from build123d import *

# Parameters (mm, degrees)
ESQUISSE1_W        = 40.5
ESQUISSE1_H        = 33.5
ESQUISSE1_W_2      = 37.5
ESQUISSE1_H_2      = 30.5
BOSS_EXTRU_1_DEPTH = 4.5
ESQUISSE2_W        = 40.5
ESQUISSE2_H        = 33.5
BOSS_EXTRU_2_DEPTH = 1.5
ESQUISSE3_R        = 1.25
BOSS_EXTRU_3_DEPTH = 5


with BuildPart() as part:
    # Esquisse1 → Boss.-Extru.1 (new body)
    with BuildSketch(Plane(origin=(0, 0, 0), x_dir=(1, 0, 0), z_dir=(0, 1, 0))):
        with Locations((18.75, 15.25)):
            Rectangle(ESQUISSE1_W, ESQUISSE1_H)
        with Locations((18.75, 15.25)):
            Rectangle(ESQUISSE1_W_2, ESQUISSE1_H_2, mode=Mode.SUBTRACT)
    extrude(amount=BOSS_EXTRU_1_DEPTH)

    # Esquisse2 → Boss.-Extru.2 (add)
    with BuildSketch(Plane.XZ):
        with Locations((18.75, -15.25)):
            Rectangle(ESQUISSE2_W, ESQUISSE2_H)
    extrude(amount=BOSS_EXTRU_2_DEPTH)

    # Esquisse3 → Boss.-Extru.3 (add)
    with BuildSketch(Plane(origin=(0, 0, 0), x_dir=(1, 0, 0), z_dir=(0, 1, 0))):
        with Locations(Location((18.75, 26.75, 0), (0, 0, 90))):
            Circle(ESQUISSE3_R)
        with Locations(Location((18.75, 3.75, 0), (0, 0, 90))):
            Circle(ESQUISSE3_R)
    extrude(amount=BOSS_EXTRU_3_DEPTH)


solid = part.part
Could you check a few things on this model? Use its own coordinates, in mm. A direction names the side the tool comes from. Coordinates: 2 decimals unless noted, no trailing zeros. Order: outer loops, then holes, each group sorted by start corner. A loop starts at its lowest first (then second) coordinate and runs counter-clockwise, first axis right, second up. Notation, with made-up numbers: (-19.75, 37.25) -> (36.25, 37.25) arc R24 ccw to (36.25, 57.25) -> close; hole circle Ø1 at (3.5, -29). An arc over 180 degrees is marked (long way). One line per item, written item: value. Start each with the question number.
1) We'd pull the mould along X, two halves only. Please class faces 3 (the flat face through (18, 2, 1.5)), 4 (the flat face through (39, 2, -15)), 5 (the cylindrical face through (19.97, 2.46, -3.48)): +X half, -X half, draft (parallel to the pull), parting line (faces both ways), or undercut.
2) Imagine slicing it at A-A on y = 1.5. List the corners of the cut face in (x, z) for me.
3) If I drill on L1, parallel to Z at x = 7.5, y = 3.25; L2, parallel to X at y = 3.5, z = -14; L3, parallel to Y at x = 13.5, z = -2, over which ranges is the centre line in solid material (lowest first)? Write a range as [from, to].
4) Imagine slicing it at B-B on x = 11. List the corners of the cut face in (y, z) for me, plus the area to 4 significant figures.
5) Which directions (+Z, -Z, +X, -X, +Y, -Y) give clear straight access to the entire face, cutting with the end or side of a thin tool? Please do faces 1 (the flat face through (0, 2, -15)), 2 (the flat face through (19, 5, -27)).
6) Imagine slicing it at D-D on x = 18.75. List the corners of the cut face in (y, z) for me, plus the area to 4 significant figures.
7) Imagine slicing it at C-C on z = -3.75. List the corners of the cut face in (x, y) for me, plus the area to 4 significant figures.
Answer list:
1. face 3: draft
1. face 4: +X half
1. face 5: undercut
2. outline: (-1.5, -32) -> (39, -32) -> (39, 1.5) -> (-1.5, 1.5) -> close; circle Ø2.5 at (18.75, -26.75); circle Ø2.5 at (18.75, -3.75); hole (0, -30.5) -> (37.5, -30.5) -> (37.5, 0) -> (0, 0) -> close
3. L1: z = [-32, -30.5], [0, 1.5]
3. L2: x = [-1.5, 0], [37.5, 39]
3. L3: y = [-1.5, 0]
4. outline: (-1.5, -32) -> (4.5, -32) -> (4.5, -30.5) -> (0, -30.5) -> (0, 0) -> (4.5, 0) -> (4.5, 1.5) -> (-1.5, 1.5) -> close
4. area: 63.75 mm2
5. face 1: +Y
5. face 2: +Z, -Z, +X, -X, +Y
6. outline: (-1.5, -32) -> (4.5, -32) -> (4.5, -30.5) -> (0, -30.5) -> (0, -28) -> (5, -28) -> (5, -25.5) -> (0, -25.5) -> (0, -5) -> (5, -5) -> (5, -2.5) -> (0, -2.5) -> (0, 0) -> (4.5, 0) -> (4.5, 1.5) -> (-1.5, 1.5) -> close
6. area: 88.75 mm2
7. outline: (-1.5, -1.5) -> (39, -1.5) -> (39, 4.5) -> (37.5, 4.5) -> (37.5, 0) -> (20, 0) -> (20, 5) -> (17.5, 5) -> (17.5, 0) -> (0, 0) -> (0, 4.5) -> (-1.5, 4.5) -> close
7. area: 86.75 mm2
